Could you check a few things on this model? Use its own coordinates, in mm. Face numbers are marked on the shaded views. A direction names the side the tool comes from. Give positions to 0.01 mm unless a question says otherwise; leave off trailing zeros. Loops run counter-clockwise (first coordinate to the right, second up) from the corner with the lowest first, then second, coordinate; pieces in that order, holes last. Notation, with made-up numbers: M 84,-12.75 L 138,-12.75 A16 ccw 138,7.25 Z; hole C 71,83.25 d10. An arc over 180 degrees is marked long. Write each question's results on one line, items separated by ' | '. Start each with the question number.
from build123d import *

# Parameters (mm, degrees)
F1_DEPTH = 50
F2_R     = 3.5
F3_DEPTH = 10
F4_R     = 3.5
F5_DEPTH = 10
F6_R     = 3.5
F7_DEPTH = 10


# Not quite as in the source:
# - a feature names something its author has since deleted; it is built from what else it names


with BuildPart() as f1:
    # F0 (on Front) → F1 (new body)
    with BuildSketch(Plane.XZ):
        Polygon((0, -6.7148432136), (25, -6.7148432136), (25, 25), (11.0791092739, 25), (11.0791092739, 12.0865814388), (0, 12.0865814388), align=None)
    extrude(amount=F1_DEPTH)

    # F2 (on face) → F3 (join)
    with BuildSketch(Plane(origin=(0, 0, 0), x_dir=(0, -1, 0), z_dir=(-1, 0, 0))):
        with Locations((13.8432676521, 3.730392782)):
            Circle(F2_R)
        with Locations((33.459926671, 3.730392782)):
            Circle(F2_R)
    extrude(amount=F3_DEPTH)

    # F4 (on face) → F5 (cut)
    with BuildSketch(Plane(origin=(0, 0, -6.7148432136), x_dir=(1, 0, 0), z_dir=(0, 0, -1))):
        with Locations((12.6557382198, 36.55)):
            Circle(F4_R)
        with Locations((13.0857451583, 13.4541578871)):
            Circle(F4_R)
    extrude(amount=-F5_DEPTH, mode=Mode.SUBTRACT)

    # F6 (on face) → F7 (join)
    with BuildSketch(Plane(origin=(11.0791092739, 0, 0), x_dir=(0, -1, 0), z_dir=(-1, 0, 0))):
        with Locations((23.5, 18.7478940934)):
            Circle(F6_R)
    extrude(amount=F7_DEPTH)


solid = f1.part
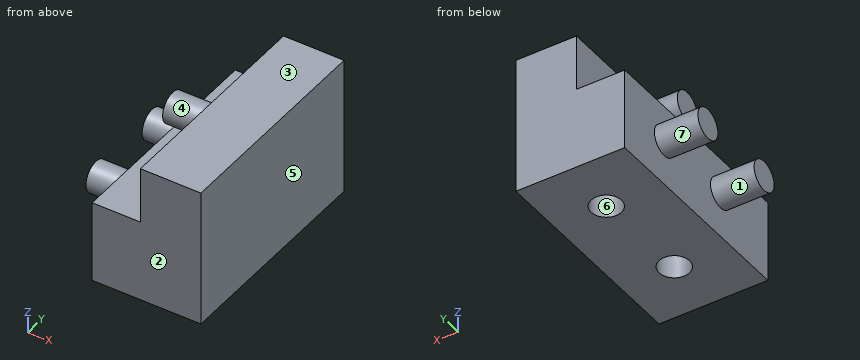
1) Which directions (+Z, -Z, +X, -X, +Y, -Y) give clear straight access to the entire face, cutting with the end or side of a thin tool? Please do the marked faces 5, 6 and 7.
2) If we section it at B-B on y = -23.5: Write out the boundary of the cut face in (x, z), plus the area to 3 significant figures.
3) Thinking about a two-plate mould opening in Z: for the marked faces 1, 2, 3 and 4, which applies, pulls with the +Z half, pulls with the -Z half, needs draft (parallel to the pull), parting line crosses it, or undercut?
4) If we section it at C-C on x = -3: Write out the boundary of the cut face in (y, z), plus the area to 3 significant figures.
5) If we section it at D-D on z = 10.5: Write out the boundary of the cut face in (x, y), plus the area to 3 significant figures.
6) I'm going to push flat-ended pins straight in: P1, Ø3.5, axis at x = 7.5, y = -17.5, coming from the +Z side; P2, Ø1.5, axis at y = -36, z = 10, coming from the -X side; P3, Ø5.5, axis at x = 13.09, y = -13.45, coming from the -Z side. Where does each tip first touch, or does it pass through?
7) If we section it at A-A on z = 2: Write out the boundary of the cut face in (x, y), plus the area to 3 significant figures.
8) Please list where these lines run through material, in increasing order: line 1 (X direction, y = -36.55, z = -3.25); line 2 (X direction, y = -28.5, z = -4); line 3 (Z direction, x = 2.5, y = -2). Write a range as from..to.
Calculated:
1) face 5: +Z, -Z, +X, +Y, -Y | face 6: -Z | face 7: -X
2) outline: M 0,-6.71 L 25,-6.71 L 25,25 L 11.08,25 L 11.08,22.25 L 1.08,22.25 L 1.08,15.25 L 11.08,15.25 L 11.08,12.09 L 0,12.09 Z | area: 720 mm2
3) face 1: parting line crosses it | face 2: needs draft | face 3: pulls with the +Z half | face 4: undercut
4) outline: C -33.46,3.73 d7; C -13.84,3.73 d7 | area: 77.0 mm2
5) outline: M 0,-50 L 25,-50 L 25,0 L 0,0 Z | area: 1,250 mm2
6) P1: stops at z = 12.09 | P2: stops at x = 0 | P3: stops at z = 3.29
7) outline: M -10,-36.5 L 0,-36.5 L 0,-50 L 25,-50 L 25,0 L 0,0 L 0,-10.8 L -10,-10.8 L -10,-16.89 L 0,-16.89 L 0,-30.42 L -10,-30.42 Z; hole C 12.66,-36.55 d7; hole C 13.09,-13.45 d7 | area: 1,290 mm2
8) line 1: x = 0..9.16, 16.16..25 | line 2: x = 0..25 | line 3: z = -6.71..12.09
